```python
from build123d import *

# Parameters (mm, degrees)
SKETCH_1_W           = 26.5
SKETCH_1_H           = 26.5
SKETCH_1_W_2         = 20.5
SKETCH_1_H_2         = 20.5
EXTRUDE_1_DEPTH      = 40
SKETCH_3_W           = 26.5
SKETCH_3_H           = 26.5
EXTRUDE_2_DEPTH      = 20
SKETCH_9_W           = 26.5
SKETCH_9_H           = 26.5
EXTRUDE_5_DEPTH      = 4
SKETCH_10_R          = 12
SKETCH_10_R_2        = 10
EXTRUDE_7_DEPTH      = 4
EXTRUDE_START        = 4
SKETCH_12_R          = 12
SKETCH_12_R_2        = 10
EXTRUDE_8_DEPTH      = 4
SKETCH_13_R          = 1.85
CUT_EXTRUDE_3_DEPTH  = 73.123591841
SKETCH_15_R          = 2.1
CUT_EXTRUDE_5_DEPTH  = 73.123591841
SKETCH_14_R          = 2.1
CUT_EXTRUDE_6_DEPTH  = 72.384959901
SKETCH_18_R          = 12
CUT_EXTRUDE_9_DEPTH  = 4
CUT_EXTRUDE_START    = 4
SKETCH_19_R          = 12
CUT_EXTRUDE_11_DEPTH = 4
FILLET_6_R           = 2
FILLET_7_R           = 2
FILLET_8_R           = 2
FILLET_9_R           = 2


with BuildPart() as part:
    # 草图1 → 凸台-拉伸1 (new body)
    with BuildSketch(Plane.XY):
        Rectangle(SKETCH_1_W, SKETCH_1_H)
        Rectangle(SKETCH_1_W_2, SKETCH_1_H_2, mode=Mode.SUBTRACT)
    extrude(amount=EXTRUDE_1_DEPTH)

    # 草图3 → 凸台-拉伸2 (add)
    with BuildSketch(Plane.XY.offset(40)):
        Rectangle(SKETCH_3_W, SKETCH_3_H)
    extrude(amount=EXTRUDE_2_DEPTH)

    # 草图9 → 凸台-拉伸5 (add)
    with BuildSketch(Plane.XY.offset(60)):
        Rectangle(SKETCH_9_W, SKETCH_9_H)
    extrude(amount=EXTRUDE_5_DEPTH)

    # 草图10 → 凸台-拉伸7 (add)
    with BuildSketch(Plane(origin=(13.25, 0, 0), x_dir=(0, 0, -1), z_dir=(1, 0, 0))):
        with Locations(Location((-50, 0, 0), (0, 0, 180))):
            Circle(SKETCH_10_R)
        with Locations((-50, 0)):
            Circle(SKETCH_10_R_2, mode=Mode.SUBTRACT)
    extrude(amount=EXTRUDE_7_DEPTH)

    # 草图12 → 凸台-拉伸8 (add)
    with BuildSketch(Plane.ZY.offset(13.25).offset(EXTRUDE_START)):
        with Locations((50, 0)):
            Circle(SKETCH_12_R)
        with Locations(Location((50, 0, 0), (0, 0, 180))):
            Circle(SKETCH_12_R_2, mode=Mode.SUBTRACT)
    extrude(amount=-EXTRUDE_8_DEPTH)

    # 草图13 → 切除-拉伸3 (cut, through all)
    with BuildSketch(Plane.ZY.offset(13.25)):
        with Locations((55.196152423, 3)):
            Circle(SKETCH_13_R)
        with Locations((50, -6)):
            Circle(SKETCH_13_R)
        with Locations((44.803847577, 3)):
            Circle(SKETCH_13_R)
    extrude(amount=-CUT_EXTRUDE_3_DEPTH, mode=Mode.SUBTRACT)

    # 草图15 → 切除-拉伸5 (cut, through all)
    with BuildSketch(Plane(origin=(13.25, 0, 0), x_dir=(0, 0, -1), z_dir=(1, 0, 0))):
        with Locations((-10, 0)):
            Circle(SKETCH_15_R)
        with Locations((-25, 0)):
            Circle(SKETCH_15_R)
    extrude(amount=-CUT_EXTRUDE_5_DEPTH, mode=Mode.SUBTRACT)

    # 草图14 → 切除-拉伸6 (cut, through all)
    with BuildSketch(Plane.XZ.offset(13.25)):
        with Locations(Location((0, 10, 0), (0, 0, 270))):
            Circle(SKETCH_14_R)
        with Locations(Location((0, 25, 0), (0, 0, 270))):
            Circle(SKETCH_14_R)
    extrude(amount=-CUT_EXTRUDE_6_DEPTH, mode=Mode.SUBTRACT)

    # 草图18 → 切除-拉伸9 (cut)
    with BuildSketch(Plane(origin=(13.25, 0, 0), x_dir=(0, 0, -1), z_dir=(1, 0, 0))):
        with Locations((-50, 0)):
            Circle(SKETCH_18_R)
    extrude(amount=CUT_EXTRUDE_9_DEPTH, mode=Mode.SUBTRACT)

    # 草图19 → 切除-拉伸11 (cut)
    with BuildSketch(Plane.ZY.offset(13.25).offset(CUT_EXTRUDE_START)):
        with Locations((50, 0)):
            Circle(SKETCH_19_R)
    extrude(amount=-CUT_EXTRUDE_11_DEPTH, mode=Mode.SUBTRACT)

    # 圆角6
    fillet_6_edges = [part.edges().sort_by_distance(p)[0] for p in [
        (0, -13.25, 64),
        (13.25, -13.25, 32),
        (-13.25, -13.25, 32),
    ]]
    fillet(fillet_6_edges, radius=FILLET_6_R)

    # 圆角7
    # the kernel refuses this fillet: 2 mm, written as the material it takes off along each edge
    with BuildSketch(Plane(origin=(11.25, -11.25, 62), x_dir=(1, 0, 0), z_dir=(0, 0, 1))) as fillet_7_piece_1_section:
        Polygon((0, 0), (FILLET_7_R, 0), (FILLET_7_R, -FILLET_7_R), (0, -FILLET_7_R), align=None)
    fillet_7_piece_1 = extrude(amount=FILLET_7_R, mode=Mode.PRIVATE)
    fillet_7_piece_1 = fillet_7_piece_1 - Plane(origin=(11.25, -11.25, 62), x_dir=(-0.7071067811865475, 0.7071067811865475, 0), z_dir=(0, 0, 1)) * Sphere(FILLET_7_R, mode=Mode.PRIVATE)
    add(fillet_7_piece_1, mode=Mode.SUBTRACT)
    with BuildSketch(Plane(origin=(13.25, 18.25, 64), x_dir=(-1, 0, 0), z_dir=(0, -1, 0))) as fillet_7_piece_2:
        with BuildLine():
            CenterArc((FILLET_7_R, FILLET_7_R), FILLET_7_R, 180, 90)
            Line((0, FILLET_7_R), (0, 0))
            Line((0, 0), (FILLET_7_R, 0))
        make_face()
    extrude(amount=29.5, mode=Mode.SUBTRACT)
    with BuildSketch(Plane(origin=(13.25, 13.25, 69), x_dir=(-1, 0, 0), z_dir=(0, 0, -1))) as fillet_7_piece_3:
        with BuildLine():
            CenterArc((FILLET_7_R, -FILLET_7_R), FILLET_7_R, 90, 90)
            Line((0, -FILLET_7_R), (0, 0))
            Line((0, 0), (FILLET_7_R, 0))
        make_face()
    extrude(amount=74, mode=Mode.SUBTRACT)

    # 圆角8
    # the kernel refuses this fillet: 2 mm, written as the material it takes off along each edge
    with BuildSketch(Plane(origin=(11.25, 11.25, 62), x_dir=(0, 1, 0), z_dir=(0, 0, 1))) as fillet_8_piece_1_section:
        Polygon((0, 0), (FILLET_8_R, 0), (FILLET_8_R, -FILLET_8_R), (0, -FILLET_8_R), align=None)
    fillet_8_piece_1 = extrude(amount=FILLET_8_R, mode=Mode.PRIVATE)
    fillet_8_piece_1 = fillet_8_piece_1 - Plane(origin=(11.25, 11.25, 62), x_dir=(-0.7071067811865475, -0.7071067811865475, 0), z_dir=(0, 0, 1)) * Sphere(FILLET_8_R, mode=Mode.PRIVATE)
    add(fillet_8_piece_1, mode=Mode.SUBTRACT)
    with BuildSketch(Plane(origin=(-18.25, 13.25, 64), x_dir=(0, -1, 0), z_dir=(1, 0, 0))) as fillet_8_piece_2:
        with BuildLine():
            CenterArc((FILLET_8_R, FILLET_8_R), FILLET_8_R, 180, 90)
            Line((0, FILLET_8_R), (0, 0))
            Line((0, 0), (FILLET_8_R, 0))
        make_face()
    extrude(amount=29.5, mode=Mode.SUBTRACT)
    with BuildSketch(Plane(origin=(-13.25, 13.25, -5), x_dir=(0, -1, 0), z_dir=(0, 0, 1))) as fillet_8_piece_3:
        with BuildLine():
            CenterArc((FILLET_8_R, FILLET_8_R), FILLET_8_R, 180, 90)
            Line((0, FILLET_8_R), (0, 0))
            Line((0, 0), (FILLET_8_R, 0))
        make_face()
    extrude(amount=74, mode=Mode.SUBTRACT)

    # 圆角9
    # the kernel refuses this fillet: 2 mm, written as the material it takes off along each edge
    with BuildSketch(Plane(origin=(-11.25, -11.25, 62), x_dir=(0, 0, 1), z_dir=(-1, 0, 0))) as fillet_9_piece_1_section:
        Polygon((0, 0), (FILLET_9_R, 0), (FILLET_9_R, -FILLET_9_R), (0, -FILLET_9_R), align=None)
    fillet_9_piece_1 = extrude(amount=FILLET_9_R, mode=Mode.PRIVATE)
    fillet_9_piece_1 = fillet_9_piece_1 - Plane(origin=(-11.25, -11.25, 62), x_dir=(0, 0.7071067811865475, -0.7071067811865475), z_dir=(-1, 0, 0)) * Sphere(FILLET_9_R, mode=Mode.PRIVATE)
    add(fillet_9_piece_1, mode=Mode.SUBTRACT)
    with BuildSketch(Plane(origin=(-11.25, 11.25, 62), x_dir=(0, 0, 1), z_dir=(-1, 0, 0))) as fillet_9_piece_2_section:
        Polygon((0, 0), (FILLET_9_R, 0), (FILLET_9_R, FILLET_9_R), (0, FILLET_9_R), align=None)
    fillet_9_piece_2 = extrude(amount=FILLET_9_R, mode=Mode.PRIVATE)
    fillet_9_piece_2 = fillet_9_piece_2 - Plane(origin=(-11.25, 11.25, 62), x_dir=(0, -0.7071067811865475, -0.7071067811865475), z_dir=(-1, 0, 0)) * Sphere(FILLET_9_R, mode=Mode.PRIVATE)
    add(fillet_9_piece_2, mode=Mode.SUBTRACT)
    with BuildSketch(Plane(origin=(-13.25, -11.25, 64), x_dir=(0, 0, -1), z_dir=(0, 1, 0))) as fillet_9_piece_3:
        with BuildLine():
            CenterArc((FILLET_9_R, -FILLET_9_R), FILLET_9_R, 90, 90)
            Line((0, -FILLET_9_R), (0, 0))
            Line((0, 0), (FILLET_9_R, 0))
        make_face()
    extrude(amount=22.5, mode=Mode.SUBTRACT)


solid = part.part
```
Geometry check sheet. Reference: the model listing, model coordinates, mm. A direction names the side the tool comes from. Round coordinates to 2 decimals unless told otherwise and drop trailing zeros. Loops run counter-clockwise (first coordinate to the right, second up) from the corner with the lowest first, then second, coordinate; pieces in that order, holes last. Notation, with made-up numbers: (71, -39.75) - (129, -39.75) arc R28 cw to (129, -13.75) - close; hole circle Ø4 at (40, 32). An arc over 180 degrees is marked (long way). Write item = value, one per line. Start each with the question number.
1. Section check A-A on z = 50. Enter the section's corners in (x, y).
2. Section check C-C on x = 0. Give the number of separate pieces and of enclosed holes in the cut face, then the cut area to 3 significant figures.
3. Mould release check, pull along Y, two halves, no side actions. Record for faces 3 (the face through (-0.16, 12.68, 63.4)), 4 (the face through (13.25, 0, 31)), 5 (the face through (-11.729, 0.631, 22.997)): released by +Y, released by -Y, zero draft, split by the parting line, or undercut.
4. Section check D-D on z = 25. Enter the section's corners in (x, y).
5. Section check B-B on y = 0. Enter the section's corners in (x, z), then the cut area to 3 significant figures.
6. Set-up check for faces 1 (the face through (0, 10.25, 20)), 2 (the face through (0.09, -11.77, 12.1)): record each of +Z, -Z, +X, -X, +Y, -Y from which the full face is reachable in a straight line by a thin tool's end or side.
7. Thickness scan on line 1 (X direction, y = -6, z = 12.5); line 2 (Z direction, x = 2.75, y = 4.25). Record the ranges inside material, lowest first.
8. Depth check by flat-ended pin: pin 1 (10 mm diameter, centred on x = -1.5, y = 3.5, fed in from -Z). Enter the tip coordinate at first touch or a pass-through.
Working result:
q1.outline = (-13.25, -11.25) arc R2 ccw to (-11.25, -13.25) - (11.25, -13.25) arc R2 ccw to (13.25, -11.25) - (13.25, -7.85) - (-13.25, -7.85) - close; (-13.25, -4.15) - (13.25, -4.15) - (13.25, 11.25) arc R2 ccw to (11.25, 13.25) - (-11.25, 13.25) arc R2 ccw to (-13.25, 11.25) - close
q2.separate_pieces = 5
q2.enclosed_holes = 3
q2.area = 792 mm^2
q3.face_3 = released by +Y
q3.face_4 = zero draft
q3.face_5 = undercut
q4.outline = (-13.25, -11.25) arc R2 ccw to (-11.25, -13.25) - (-2.1, -13.25) - (-2.1, -10.25) - (-10.25, -10.25) - (-10.25, -2.1) - (-13.25, -2.1) - close; (-13.25, 2.1) - (-10.25, 2.1) - (-10.25, 10.25) - (-2.1, 10.25) - (-2.1, 13.25) - (-11.25, 13.25) arc R2 ccw to (-13.25, 11.25) - close; (2.1, -13.25) - (11.25, -13.25) arc R2 ccw to (13.25, -11.25) - (13.25, -2.1) - (10.25, -2.1) - (10.25, -10.25) - (2.1, -10.25) - close; (2.1, 10.25) - (10.25, 10.25) - (10.25, 2.1) - (13.25, 2.1) - (13.25, 11.25) arc R2 ccw to (11.25, 13.25) - (2.1, 13.25) - close
q5.outline = (-13.25, 0) - (-10.25, 0) - (-10.25, 7.9) - (-13.25, 7.9) - close; (-13.25, 12.1) - (-10.25, 12.1) - (-10.25, 22.9) - (-13.25, 22.9) - close; (-13.25, 27.1) - (-10.25, 27.1) - (-10.25, 40) - (10.25, 40) - (10.25, 27.1) - (13.25, 27.1) - (13.25, 62) arc R2 ccw to (11.25, 64) - (-11.25, 64) arc R2 ccw to (-13.25, 62) - close; (10.25, 0) - (13.25, 0) - (13.25, 7.9) - (10.25, 7.9) - close; (10.25, 12.1) - (13.25, 12.1) - (13.25, 22.9) - (10.25, 22.9) - close
q5.area = 824 mm^2
q6.face_1 = -Z
q6.face_2 = +Y, -Y
q7.line_1 = -13.25 to -10.25, 10.25 to 13.25
q7.line_2 = 40 to 43.44, 46.17 to 53.83, 56.56 to 64
q8.pin_1 = 40
